Autodesk Inventor part; units mm, degrees
ref_plane "YZ Plane" through (0, 0, 0) normal (1, 0, 0) x (0, 1, 0)
ref_plane "XZ Plane" through (0, 0, 0) normal (0, 1, 0) x (-1, 0, 0)
ref_plane "XY Plane" through (0, 0, 0) normal (0, 0, 1) x (1, 0, 0)
sketch "Sketch1" plane through (0, 0, 0) normal (0, 1, 0) x (-1, 0, 0)
  line L0 (-10, 10) -> (10, 10)
  line L1 (10, 10) -> (10, -10)
  line L2 (10, -10) -> (-10, -10)
  line L3 (-10, -10) -> (-10, 10)
  line L4 (-10, 10) -> (10, -10) construction
  line L5 (10, 10) -> (-10, -10) construction
  point P0 (0, 0)
  dimension "d0" = 20
  dimension "d1" = 20
extrude "Extrusion1" add sketch "Sketch1" along normal blind 5
sketch "Sketch3" plane through (0, 0, 0) normal (0, -1, 0) x (1, 0, 0)
  line L0 (0, 4.6188) -> (4, 2.3094)
  line L1 (4, 2.3094) -> (4, -2.3094)
  line L2 (4, -2.3094) -> (0, -4.6188)
  line L3 (0, -4.6188) -> (-4, -2.3094)
  line L4 (-4, -2.3094) -> (-4, 2.3094)
  line L5 (-4, 2.3094) -> (0, 4.6188)
  line L6 (10, 10) -> (10, -10)
  point P0 (0, 0)
  point P1 (0, 0)
  point P2 (-4, 0)
  dimension "d7" = 8
extrude "Extrusion3" cut sketch "Sketch3" against normal blind 2
sketch "Sketch2" plane through (0, 0, 0) normal (0, -1, 0) x (1, 0, 0)
  circle A0 centre (0, 0) radius 2.75
  dimension "d4" = 5.5
extrude "Extrusion2" cut sketch "Sketch2" against normal blind 22.5
sketch "Sketch4" plane through (0, 5, 0) normal (0, 1, 0) x (1, 0, 0)
  line L0 (1.5, 6) -> (-1.5, 6)
  line L1 (-1.5, 6) -> (-1.5, -6)
  line L2 (-1.5, -6) -> (1.5, -6)
  line L3 (1.5, -6) -> (1.5, 6)
  circle A0 centre (0, 0) radius 2.75
  line L4 (1.5, 6) -> (-1.5, -6) construction
  line L5 (-1.5, 6) -> (1.5, -6) construction
  dimension "d10" = 6
  dimension "d11" = 3
extrude "Extrusion4" add sketch "Sketch4" along normal blind 20 contours L3 A0 L1 L0 | L3 A0 L1 | L3 L2 L1 A0
sketch "Sketch5" plane through (0, 2, 0) normal (0, -1, 0) x (1, 0, 0)
  circle A0 centre (0, 0) radius 2.75
  dimension "d14" = 5.5
extrude "Extrusion5" cut sketch "Sketch5" against normal blind 10
fillet "Fillet1" radius 10 4 edges at (-10, 2.5, -10) (-10, 2.5, 10) (10, 2.5, -10) (10, 2.5, 10)
fillet "Fillet2" radius 5 2 edges at (0, 25, -6) (0, 25, 6)
sketch "Sketch6" plane through (1.5, 5, 6) normal (1, 0, 0) x (0, 0, -1)
  line L0 (6, 19.4737) -> (10, 17.1643)
  line L1 (10, 17.1643) -> (10, 12.5455)
  line L2 (10, 12.5455) -> (6, 10.2361)
  line L3 (6, 10.2361) -> (2, 12.5455)
  line L4 (2, 12.5455) -> (2, 17.1643)
  line L5 (2, 17.1643) -> (6, 19.4737)
  line L6 (12, 0) -> (12, 15)
  point P0 (6, -5)
  point P1 (6, 14.8549)
  dimension "d21" = 8
extrude "Extrusion6" cut sketch "Sketch6" against normal blind 2
sketch "Sketch7" plane through (-0.5, 5, 6) normal (1, 0, 0) x (0, 0, -1)
  circle A0 centre (6, 14.75) radius 2.75
  line L0 (12, 0) -> (12, 15)
  line L1 (5, 20) -> (7, 20)
  point P0 (6, -5)
  point P1 (6, 20)
  dimension "d24" = 5.5
  dimension "d25" = 6
  dimension "d26" = 5.25
extrude "Extrusion7" cut sketch "Sketch7" against normal blind 40.5
properties part number "J2"
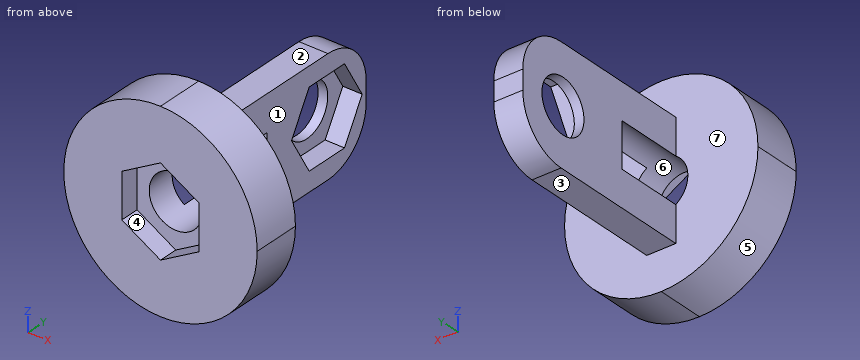
Can you work these out from the model? Positions are in its coordinate system, mm. Face numbers are marked on the shaded views. A direction names the side the tool comes from. Round coordinates to 2 decimals unless told otherwise and drop trailing zeros. Loops run counter-clockwise (first coordinate to the right, second up) from the corner with the lowest first, then second, coordinate; pieces in that order, holes last. Notation, with made-up numbers: M 68.25,-17 L 104.25,-17 A17 ccw 104.25,-7 Z; hole C 80.25,78 d11. An arc over 180 degrees is marked long. Answer as a JSON object with one key per item and string values. Group by question number.
Q1. We'd pull the mould along Z, two halves only. Please class the marked faces 5, 6 and 7: +Z half, -Z half, draft (parallel to the pull), parting line (faces both ways), or undercut.
Q2. Will these pins go through, and if not, where does the flat tip stop? pin 1 (0.9 mm diameter, centred on x = -0.5, y = 10, fed in from +Z); pin 2 (2 mm diameter, centred on x = 0.5, y = 21, fed in from -Z); pin 3 (3.5 mm diameter, centred on x = 0, z = 0, fed in from -Y); pin 4 (9 mm diameter, centred on x = -0.5, z = -0.5, fed in from -Y).
Q3. Imagine slicing it at A-A, the plane y = 8.5. Please give me the cut outline in (x, z).
Q4. Imagine slicing it at C-C, the plane z = -7.5. Please give me the cut outline in (x, y).
Q5. Imagine slicing it at B-B, the plane y = 16.25. Please give me the cut outline in (x, z).
Q6. Please list where these lines run through material, in increasing order: L1, parallel to Y at x = -1, z = 0; L2, parallel to Y at x = 3.25, z = -0.75; L3, parallel to Y at x = -5.75, z = 7.5.
Q7. Imagine slicing it at D-D, the plane x = -4.5. Please give me the cut outline in (y, z).
Q8. On a 3-axis mill with a long thin cutter (end or side, diameter ignored), from which of +Z, -Z, +X, -X, +Y, -Y can I reach the whole of each face in a straight line? I mean the marked faces 1, 2, 3 and 4. Say none if no direction works.
Findings:
{
 "1": {"face 5": "-Z half", "face 6": "undercut", "face 7": "draft"},
 "2": {"pin 1": "stops at z = 6", "pin 2": "stops at z = -6", "pin 3": "stops at y = 12", "pin 4": "stops at y = 0"},
 "3": {"outline": "M -1.5,-6 L 1.5,-6 L 1.5,-2.3 A2.75 cw -1.5,-2.3 Z; M -1.5,2.3 A2.75 cw 1.5,2.3 L 1.5,6 L -1.5,6 Z"},
 "4": {"outline": "M -6.61,0 L 6.61,0 L 6.61,5 L -6.61,5 Z"},
 "5": {"outline": "M -1.5,-6 L 1.5,-6 L 1.5,-1.76 L -0.5,-1.76 L -0.5,1.76 L 1.5,1.76 L 1.5,6 L -1.5,6 Z"},
 "6": {"L1": "y = 12 to 17, 22.5 to 25", "L2": "y = 2 to 5", "L3": "y = 0 to 5"},
 "7": {"outline": "M 0,-8.93 L 5,-8.93 L 5,8.93 L 0,8.93 Z"},
 "8": {"face 1": "+Z, -Z, +X, +Y", "face 2": "+Z, +X, -X, +Y", "face 3": "-Z, +X, -X, +Y", "face 4": "-Y"}
}
